The model under review builds one solid part; all positions refer to its coordinate system, in mm. Give positions to 0.01 mm unless a question says otherwise; leave off trailing zeros. Loops run counter-clockwise (first coordinate to the right, second up) from the corner with the lowest first, then second, coordinate; pieces in that order, holes last. Notation, with made-up numbers: M 52,41.5 L 93,41.5 A33 ccw 93,75.5 Z; hole C 76.25,21.5 d1. An arc over 180 degrees is marked long. Return JSON: item names as keys, results as strings.
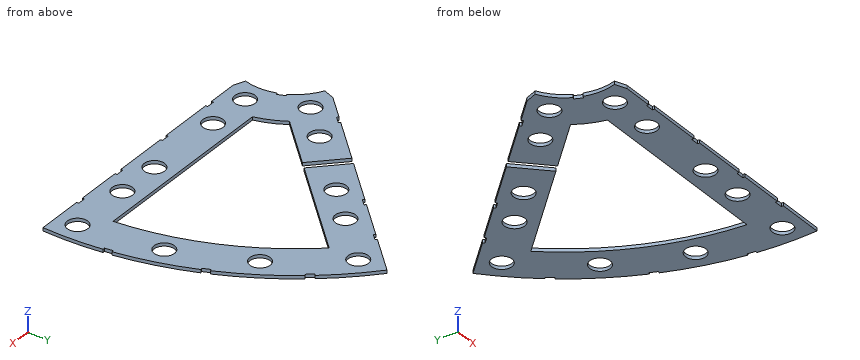
```python
from build123d import *

# Parameters (mm, degrees)
BOSS_EXTRUDE1_DEPTH = 1
SKETCH2_R           = 3.175
CUT_EXTRUDE1_DEPTH  = 2
SKETCH3_W           = 2.54
SKETCH3_H           = 0.635
CUT_EXTRUDE2_DEPTH  = 2


with BuildPart() as part:
    # Sketch1 → Boss-Extrude1 (new body)
    with BuildSketch(Plane.XY):
        with BuildLine():
            Line((67.21146711, 76.191723231), (8.696654013, 17.676910134))
            Line((8.696654013, 17.676910134), (7.228954972, 14.133571205))
            ThreePointArc((7.228954972, 14.133571205), (14.666587579, 6.075099489), (15.105587123, -4.88230096))
            Line((15.105587123, -4.88230096), (18.648926052, -6.35))
            Line((18.648926052, -6.35), (101.401368334, -6.35))
            ThreePointArc((101.401368334, -6.35), (93.866160503, 38.880636728), (67.21146711, 76.191723231))
        make_face()
        with BuildLine():
            Line((88.672924278, 6.35), (27.86051193, 6.35))
            ThreePointArc((27.86051193, 6.35), (26.399857642, 10.93517908), (24.190484974, 15.210228852))
            Line((24.190484974, 15.210228852), (67.191354125, 58.211098004))
            ThreePointArc((67.191354125, 58.211098004), (82.13289044, 34.020557137), (88.672924278, 6.35))
        make_face(mode=Mode.SUBTRACT)
    extrude(amount=BOSS_EXTRUDE1_DEPTH)

    # Sketch2 → Cut-Extrude1 (cut, through all)
    with BuildSketch(Plane.XY.offset(1)):
        with Locations((22.225, 0)):
            Circle(SKETCH2_R)
        with Locations((36.195, 0)):
            Circle(SKETCH2_R)
        with Locations((61.722, 0)):
            Circle(SKETCH2_R)
        with Locations((75.692, 0)):
            Circle(SKETCH2_R)
        with Locations((95.25, 0)):
            Circle(SKETCH2_R)
        with Locations((15.715448212, 15.715448212)):
            Circle(SKETCH2_R)
        with Locations((25.593729945, 25.593729945)):
            Circle(SKETCH2_R)
        with Locations((43.644044748, 43.644044748)):
            Circle(SKETCH2_R)
        with Locations((53.522326482, 53.522326482)):
            Circle(SKETCH2_R)
        with Locations((92.004434954, 24.652514046)):
            Circle(SKETCH2_R)
        with Locations((82.48891971, 47.625)):
            Circle(SKETCH2_R)
        with Locations((67.351920908, 67.351920908)):
            Circle(SKETCH2_R)
    extrude(amount=-CUT_EXTRUDE1_DEPTH, mode=Mode.SUBTRACT)

    # Sketch3 → Cut-Extrude2 (cut, through all)
    with BuildSketch(Plane.XY.offset(1)):
        Polygon((15.266435406, 24.246691527), (17.06248663, 26.042742751), (17.511499436, 25.593729945), (15.715448212, 23.797678721), align=None)
        Polygon((44.991083167, 53.971339288), (43.195031942, 52.175288063), (43.644044748, 51.726275257), (45.440095973, 53.522326482), align=None)
        with Locations((29.21, -6.0325)):
            Rectangle(SKETCH3_W, SKETCH3_H)
        with Locations((68.707, -6.0325)):
            Rectangle(SKETCH3_W, SKETCH3_H)
        Polygon((29.230733674, 38.210989795), (31.026784898, 40.007041019), (40.007041019, 31.026784898), (38.210989795, 29.230733674), align=None)
        Polygon((56.845021246, 65.825277367), (55.048970022, 64.029226143), (55.497982828, 63.580213337), (57.294034052, 65.376264561), align=None)
        with Locations((48.9585, -6.0325)):
            Rectangle(SKETCH3_W, SKETCH3_H)
        with Locations((85.471, -6.0325)):
            Rectangle(SKETCH3_W, SKETCH3_H)
        Polygon((99.935462164, 14.437711971), (100.266998693, 11.919442024), (101.526133667, 12.085210288), (101.194597138, 14.603480236), align=None)
        Polygon((93.765504959, 37.464305742), (94.938831965, 37.950313702), (93.966816047, 40.296967714), (92.793489041, 39.810959755), align=None)
        Polygon((79.327792988, 62.471156422), (80.874047017, 60.456038938), (81.88160576, 61.229165953), (80.33535173, 63.244283437), align=None)
        Polygon((13.593916116, 7.005422516), (14.565932035, 4.658768503), (15.739259041, 5.144776462), (14.767243123, 7.491430475), align=None)
    extrude(amount=-CUT_EXTRUDE2_DEPTH, mode=Mode.SUBTRACT)


solid = part.part
```
1) Consider section C-C on z = 0.7. Count the separate pieces of the cut face and the enclosed holes in it, then the cut area to 3 significant figures.
From the geometry:
{"separate pieces": "1", "enclosed holes": "12", "area": "2,600 mm²"}
2) Wall thickness on L1, parallel to Y at x = 66.5, z = 0.15; L2, parallel to X at y = 51.5, z = 0.5; L3, parallel to Y at x = 24.5, z = 0.2: over which ranges is each line inside the solid? List them lowest first. Write a range as from..to.
From the geometry:
{"L1": "-6.35..6.35, 57.52..64.29, 70.41..75.48", "L2": "42.52..51.07, 55.97..60.48, 72.46..87.58", "L3": "-6.35..-2.21, 2.21..14.71, 15.52..22.61, 28.57..33.48"}
3) Insertion check: pin 1 (0.5 mm diameter, centred on y = -6, z = 0.5, fed in from +X). The pin has a flat end and moves straight along its axis. Give the tip position at first contact, or say it passes through.
From the geometry:
{"pin 1": "x = 101.44"}
4) Consider section B-B on x = 68.5. Write out the cut boundary in (y, z) (3 decimals), then the cut area to 3 significant figures.
From the geometry:
{"outline": "M -5.715,0 L 6.35,0 L 6.35,1 L -5.715,1 Z; M 56.665,0 L 64.392,0 L 64.392,1 L 56.665,1 Z; M 70.312,0 L 75.035,0 L 75.035,1 L 70.312,1 Z", "area": "24.5 mm²"}
5) Consider section A-A on y = 0. Write out the cut boundary in (x, z) (3 decimals).
From the geometry:
{"outline": "M 15.875,0 L 19.05,0 L 19.05,1 L 15.875,1 Z; M 25.4,0 L 33.02,0 L 33.02,1 L 25.4,1 Z; M 39.37,0 L 58.547,0 L 58.547,1 L 39.37,1 Z; M 64.897,0 L 72.517,0 L 72.517,1 L 64.897,1 Z; M 78.867,0 L 92.075,0 L 92.075,1 L 78.867,1 Z; M 98.425,0 L 101.6,0 L 101.6,1 L 98.425,1 Z"}
